from build123d import *

# Parameters (mm, degrees)
BASE_R                                     = 100
BASE_CIRCLE_DEPTH                          = 10
VERT_START                                 = 5
CUTOUT_W                                   = 4.6
CUTOUT_H                                   = 20
CUTOUT_W_2                                 = 0.4
CUTOUT_W_3                                 = 4.5
CUTOUT_H_2                                 = 15
VERT_SUPPORT_DEPTH                         = 137.774468788
F_1_START                                  = 23.05
F_1_OFFSET_FOR_VERT_SUPPORT_OUTLINE_W      = 5.1
F_1_OFFSET_FOR_VERT_SUPPORT_OUTLINE_H      = 20.2
F_1_OFFSET_FOR_VERT_SUPPORT_DEPTH          = 5.2
F_1_START_2                                = -30.1
F_1_OFFSET_FOR_VERT_SUPPORT_2_OUTLINE_W    = 5.1
F_1_OFFSET_FOR_VERT_SUPPORT_2_OUTLINE_H    = 15.2
F_1_OFFSET_FOR_VERT_SUPPORT_2_DEPTH        = 4.7
CUTOUT_3_W                                 = 20
CUTOUT_3_H                                 = 40
SERVO_CUTOUT_DEPTH                         = 142.774468788
SKETCH4_W                                  = 20
SKETCH4_H                                  = 54
SERVO_REST_DEPTH                           = 2.4
SERVO_SLANT_1_SIZE                         = 5.3
SERVO_SLANT_1_SIZE2                        = 1.7
SERVO_SLANT_2_SIZE                         = 1.7
SERVO_SLANT_2_SIZE2                        = 5.3
F_15_START                                 = -52.15
F_15_SERVO_PRINT_OFFSET_DEPTH              = 20.3
SKETCH6_R                                  = 2.25
M4_THREAD_CLEARANCE_WIGGLE_ROOM_DEPTH      = 142.774468788
SKETCH6_3_R                                = 3.75
M4_SOCKET_HEAD_CLEARANCE_WIGGLE_ROOM_DEPTH = 2
SKETCH5_R                                  = 10
SKETCH5_R_2                                = 7
CENTRAL_AXLE_HEAD_CUTOUT_DEPTH             = 5
SKETCH5_3_R                                = 7
AXLE_BODY_CUTOUT_DEPTH                     = 142.774468788
F_15_OFFSET_AXLE_BY                        = 0.2
F_15_OFFSET_AXLE_2_BY                      = 0.2
F_15_OFFSET_AXLE_3_BY                      = 0.2
SKETCH8_W                                  = 124.3
SKETCH8_H                                  = 94.3
INTERSECT_TOOL_DEPTH                       = 10
CORNER_CHAMFER_SIZE                        = 10
EDGE_CHAMFER_SIZE                          = 5


# Read off the part's stored shape, not the designer's step: .1 Offset for vert support, .15 Servo Print Offset
with BuildPart() as part:
    # Base → Base Circle (new body)
    with BuildSketch(Plane(origin=(0, 0, 0), x_dir=(1, 0, 0), z_dir=(0, 1, 0))):
        with Locations(Location((0, 0, 0), (0, 0, 270))):
            Circle(BASE_R)
    extrude(amount=BASE_CIRCLE_DEPTH)

    # Cutout → Vert Support (cut, through all)
    with BuildSketch(Plane(origin=(0, 0, 0), x_dir=(1, 0, 0), z_dir=(0, 1, 0)).offset(VERT_START)):
        with Locations((25.45, 0)):
            Rectangle(CUTOUT_W, CUTOUT_H)
        with Locations((27.95, 0)):
            Rectangle(CUTOUT_W_2, CUTOUT_H)
        with Locations((-27.75, 0)):
            Rectangle(CUTOUT_W_3, CUTOUT_H_2)
    extrude(amount=VERT_SUPPORT_DEPTH, mode=Mode.SUBTRACT)

    # .1 Offset for vert support outline → .1 Offset for vert support (cut)
    with BuildSketch(Plane.YZ.offset(F_1_START)):
        with Locations((7.45, 0)):
            Rectangle(F_1_OFFSET_FOR_VERT_SUPPORT_OUTLINE_W, F_1_OFFSET_FOR_VERT_SUPPORT_OUTLINE_H)
    extrude(amount=F_1_OFFSET_FOR_VERT_SUPPORT_DEPTH, mode=Mode.SUBTRACT)

    # 1 Offset for vert support 2 outline → 1 Offset for vert support 2 (cut)
    with BuildSketch(Plane.YZ.offset(F_1_START_2)):
        with Locations((7.45, 0)):
            Rectangle(F_1_OFFSET_FOR_VERT_SUPPORT_2_OUTLINE_W, F_1_OFFSET_FOR_VERT_SUPPORT_2_OUTLINE_H)
    extrude(amount=F_1_OFFSET_FOR_VERT_SUPPORT_2_DEPTH, mode=Mode.SUBTRACT)

    # Cutout<3> → Servo cutout (cut, through all)
    with BuildSketch(Plane(origin=(0, 0, 0), x_dir=(1, 0, 0), z_dir=(0, 1, 0))):
        with Locations((-42, 10)):
            Rectangle(CUTOUT_3_W, CUTOUT_3_H)
    extrude(amount=SERVO_CUTOUT_DEPTH, mode=Mode.SUBTRACT)

    # Sketch4 → Servo rest (cut)
    with BuildSketch(Plane.XZ.offset(-10)):
        with Locations((-42, -10)):
            Rectangle(SKETCH4_W, SKETCH4_H)
    extrude(amount=SERVO_REST_DEPTH, mode=Mode.SUBTRACT)

    # Servo Slant 1
    servo_slant_1_edges = [part.edges().sort_by_distance(p)[0] for p in [
        (-42, 7.6, -30),
    ]]
    servo_slant_1_side = [part.faces().sort_by_distance(p)[0] for p in [
        (-42, 7.6, -33.5),
    ]]
    chamfer(servo_slant_1_edges, length=SERVO_SLANT_1_SIZE, length2=SERVO_SLANT_1_SIZE2, reference=servo_slant_1_side[0])

    # Servo Slant 2
    servo_slant_2_edges = [part.edges().sort_by_distance(p)[0] for p in [
        (-42, 7.6, 10),
    ]]
    servo_slant_2_side = [part.faces().sort_by_distance(p)[0] for p in [
        (-42, 3.8, 10),
    ]]
    chamfer(servo_slant_2_edges, length=SERVO_SLANT_2_SIZE, length2=SERVO_SLANT_2_SIZE2, reference=servo_slant_2_side[0])

    # .15 Servo Print Offset outline → .15 Servo Print Offset (cut)
    with BuildSketch(Plane.YZ.offset(F_15_START)):
        Polygon((10, 17.15), (7.45, 17.15), (7.45, 15.323467766), (5.742472603, 10), (0, 10), (0, -30), (5.742472603, -30), (7.45, -35.323467766), (7.45, -37.15), (10, -37.15), align=None)
    extrude(amount=F_15_SERVO_PRINT_OFFSET_DEPTH, mode=Mode.SUBTRACT)

    # Sketch6 → M4 Thread Clearance + wiggle room (cut, through all)
    with BuildSketch(Plane.XZ):
        with Locations(Location((-47, -34.5, 0), (0, 0, 270))):
            Circle(SKETCH6_R)
        with Locations(Location((-37, -34.5, 0), (0, 0, 270))):
            Circle(SKETCH6_R)
        with Locations(Location((-37, 14.5, 0), (0, 0, 270))):
            Circle(SKETCH6_R)
        with Locations(Location((-47, 14.5, 0), (0, 0, 270))):
            Circle(SKETCH6_R)
    extrude(amount=-M4_THREAD_CLEARANCE_WIGGLE_ROOM_DEPTH, mode=Mode.SUBTRACT)

    # Sketch6<3> → M4 Socket Head Clearance + wiggle room (cut)
    with BuildSketch(Plane.XZ):
        with Locations(Location((-47, -34.5, 0), (0, 0, 270))):
            Circle(SKETCH6_3_R)
        with Locations(Location((-37, -34.5, 0), (0, 0, 270))):
            Circle(SKETCH6_3_R)
        with Locations(Location((-37, 14.5, 0), (0, 0, 270))):
            Circle(SKETCH6_3_R)
        with Locations(Location((-47, 14.5, 0), (0, 0, 270))):
            Circle(SKETCH6_3_R)
    extrude(amount=-M4_SOCKET_HEAD_CLEARANCE_WIGGLE_ROOM_DEPTH, mode=Mode.SUBTRACT)

    # Sketch5 → Central Axle Head cutout (cut)
    with BuildSketch(Plane(origin=(0, 10, 0), x_dir=(1, 0, 0), z_dir=(0, 1, 0))):
        with Locations(Location((0, 0, 0), (0, 0, 270))):
            Circle(SKETCH5_R)
        with Locations(Location((0, 0, 0), (0, 0, 270))):
            Circle(SKETCH5_R_2, mode=Mode.SUBTRACT)
    extrude(amount=-CENTRAL_AXLE_HEAD_CUTOUT_DEPTH, mode=Mode.SUBTRACT)

    # Sketch5<3> → Axle Body cutout (cut, through all)
    with BuildSketch(Plane(origin=(0, 10, 0), x_dir=(1, 0, 0), z_dir=(0, 1, 0))):
        with Locations(Location((0, 0, 0), (0, 0, 270))):
            Circle(SKETCH5_3_R)
    extrude(amount=-AXLE_BODY_CUTOUT_DEPTH, mode=Mode.SUBTRACT)

    # .15 Offset, Axle: a face moved inward by 0.2
    extrude(part.faces().sort_by_distance((0, 5, 8))[0], amount=F_15_OFFSET_AXLE_BY, dir=(0, -1, 0), mode=Mode.SUBTRACT)

    # 15 Offset_ Axle 2: a curved face moved inward by 0.2
    add(Solid.thicken(part.faces().sort_by_distance((0, 2.5, -7))[0], -F_15_OFFSET_AXLE_2_BY), mode=Mode.SUBTRACT)

    # 15 Offset_ Axle 3: a curved face moved inward by 0.2
    add(Solid.thicken(part.faces().sort_by_distance((0, 7.5, -10))[0], -F_15_OFFSET_AXLE_3_BY), mode=Mode.SUBTRACT)


with BuildPart() as body_2:
    # Sketch8 → Intersect Tool (new body)
    with BuildSketch(Plane(origin=(0, 10, 0), x_dir=(1, 0, 0), z_dir=(0, 1, 0))):
        Rectangle(SKETCH8_W, SKETCH8_H)
    extrude(amount=-INTERSECT_TOOL_DEPTH)


with BuildPart() as part_1:
    add(part.part)

    # Intersect with tool: intersect body 2
    add(body_2.part, mode=Mode.INTERSECT)

    # Corner Chamfer
    corner_chamfer_edges = [part_1.edges().sort_by_distance(p)[0] for p in [
        (62.15, 5, -47.15),
        (62.15, 5, 47.15),
        (-62.15, 5, 47.15),
        (-62.15, 5, -47.15),
    ]]
    chamfer(corner_chamfer_edges, length=CORNER_CHAMFER_SIZE)

    # Edge Chamfer
    edge_chamfer_edges = [part_1.edges().sort_by_distance(p)[0] for p in [
        (-57.15, 10, -42.15),
        (0, 10, -47.15),
        (57.15, 10, -42.15),
        (62.15, 10, 0),
        (57.15, 10, 42.15),
        (0, 10, 47.15),
        (-57.15, 10, 42.15),
        (-62.15, 10, 0),
        (-57.15, 0, -42.15),
        (0, 0, -47.15),
        (57.15, 0, -42.15),
        (62.15, 0, 0),
        (57.15, 0, 42.15),
        (-62.15, 0, 0),
        (-57.15, 0, 42.15),
        (0, 0, 47.15),
    ]]
    chamfer(edge_chamfer_edges, length=EDGE_CHAMFER_SIZE - 0.0001)  # a hair under: the kernel refuses the full size


solid = part_1.part
Check sheet for the modelled part. Datum: model origin and axes. Units: mm. A direction names the side the tool comes from. Round coordinates to 2 decimals unless told otherwise and drop trailing zeros.
1. Scan lines: probe 1 along X at (y, z) = (6.5, -9); probe 2 along X at (y, z) = (0.8, -34.5); probe 3 along Z at (x, y) = (-47, 4.6). Record each from-to range of solid material in increasing order.
2. Gauge pin test, flat ends, axial feed: pin 1 Ø5.5 at (y, z) = (8, 2) entering from +X; pin 2 Ø0.9 at (x, z) = (-45, 16.5) entering from +Y; pin 3 Ø6 at (x, z) = (-37, 14.5) entering from -Y. Record the tip position at first contact, or that the pin passes through.
3. Sectioned sample at C-C on z = -3. Give the number of separate pieces and of enclosed holes in the cut face, and give its area (3 significant figures).
4. Set-up check for faces 1 (the flat face through (-28, 7, 7.6)), 2 (the cylindrical face through (-50.66, 0.99, 15.31)), 3 (the flat face through (55.337, 2.535, -40.477)): record each of +Z, -Z, +X, -X, +Y, -Y from which the full face is reachable in a straight line by a thin tool's end or side.
5. Mould release check, pull along X, two halves, no side actions. Record for faces 4 (the flat face through (59.615, 7.535, 0.52)), 5 (the flat face through (-55.477, 2.535, -40.337)), 6 (the flat face through (-42, 3, -30)), 7 (the cylindrical face through (-39.282, 0.986, 17.476)): released by +X, released by -X, zero draft, split by the parting line, or undercut.
Recorded:
1. probe 1: x = -60.65 to -52.15, -31.85 to -4.8, 4.8 to 23.05, 28.25 to 60.65
1. probe 2: x = -57.95 to -50.75, -43.25 to -40.75, -33.25 to 57.95
1. probe 3: z = -46.75 to -36.75, -32.25 to -30, 10 to 12.25, 16.75 to 46.75
2. pin 1: stops at x = 61.9
2. pin 2: stops at y = 7.45
2. pin 3: stops at y = 2
3. separate pieces: 3
3. enclosed holes: 0
3. area: 775 mm2
4. face 1: +Y
4. face 2: -Y
4. face 3: -Z, +X, -Y
5. face 4: released by +X
5. face 5: released by -X
5. face 6: undercut
5. face 7: undercut
